```python
from build123d import *

# Parameters (mm, degrees)
SKETCH_1_R        = 110
SKETCH_1_R_2      = 3
SKETCH_1_R_3      = 90
EXTRUDE_1_DEPTH   = 10
SKETCH_1_R_4      = 80
SKETCH_1_R_5      = 75
EXTRUDE_1_2_DEPTH = 10
SKETCH_1_3_R      = 90
SKETCH_1_3_R_2    = 80
SKETCH_1_3_R_3    = 75
EXTRUDE_2_DEPTH   = 5
SKETCH_2_R        = 90
SKETCH_2_R_2      = 80
EXTRUDE_4_DEPTH   = 5


with BuildPart() as part:
    # Sketch 1 → Extrude 1 (new body)
    with BuildSketch(Plane(origin=(0, 0, 0), x_dir=(1, 0, 0), z_dir=(0, 1, 0))):
        with Locations(Location((0, 0, 0), (0, 0, 270))):
            Circle(SKETCH_1_R)
        with Locations(Location((-38.268343237, 92.387953251, 0), (0, 0, 270))):
            Circle(SKETCH_1_R_2, mode=Mode.SUBTRACT)
        with Locations(Location((-70.710678119, 70.710678119, 0), (0, 0, 270))):
            Circle(SKETCH_1_R_2, mode=Mode.SUBTRACT)
        with Locations(Location((-92.387953251, 38.268343237, 0), (0, 0, 270))):
            Circle(SKETCH_1_R_2, mode=Mode.SUBTRACT)
        with Locations(Location((-100, 0, 0), (0, 0, 270))):
            Circle(SKETCH_1_R_2, mode=Mode.SUBTRACT)
        with Locations(Location((-92.387953251, -38.268343237, 0), (0, 0, 270))):
            Circle(SKETCH_1_R_2, mode=Mode.SUBTRACT)
        with Locations(Location((-70.710678119, -70.710678119, 0), (0, 0, 270))):
            Circle(SKETCH_1_R_2, mode=Mode.SUBTRACT)
        with Locations(Location((-38.268343237, -92.387953251, 0), (0, 0, 270))):
            Circle(SKETCH_1_R_2, mode=Mode.SUBTRACT)
        with Locations(Location((0, -100, 0), (0, 0, 270))):
            Circle(SKETCH_1_R_2, mode=Mode.SUBTRACT)
        with Locations(Location((38.268343237, -92.387953251, 0), (0, 0, 270))):
            Circle(SKETCH_1_R_2, mode=Mode.SUBTRACT)
        with Locations(Location((70.710678119, -70.710678119, 0), (0, 0, 270))):
            Circle(SKETCH_1_R_2, mode=Mode.SUBTRACT)
        with Locations(Location((92.387953251, -38.268343237, 0), (0, 0, 270))):
            Circle(SKETCH_1_R_2, mode=Mode.SUBTRACT)
        with Locations(Location((100, 0, 0), (0, 0, 270))):
            Circle(SKETCH_1_R_2, mode=Mode.SUBTRACT)
        with Locations(Location((92.387953251, 38.268343237, 0), (0, 0, 270))):
            Circle(SKETCH_1_R_2, mode=Mode.SUBTRACT)
        with Locations(Location((70.710678119, 70.710678119, 0), (0, 0, 270))):
            Circle(SKETCH_1_R_2, mode=Mode.SUBTRACT)
        with Locations(Location((38.268343237, 92.387953251, 0), (0, 0, 270))):
            Circle(SKETCH_1_R_2, mode=Mode.SUBTRACT)
        with Locations(Location((0, 100, 0), (0, 0, 270))):
            Circle(SKETCH_1_R_2, mode=Mode.SUBTRACT)
        with Locations(Location((0, 0, 0), (0, 0, 270))):
            Circle(SKETCH_1_R_3, mode=Mode.SUBTRACT)
    extrude(amount=EXTRUDE_1_DEPTH)



with BuildPart() as body_2:
    # Sketch 1 → Extrude 1 2 (new body)
    with BuildSketch(Plane(origin=(0, 0, 0), x_dir=(1, 0, 0), z_dir=(0, 1, 0))):
        with Locations(Location((0, 0, 0), (0, 0, 270))):
            Circle(SKETCH_1_R_4)
        with Locations(Location((0, 0, 0), (0, 0, 270))):
            Circle(SKETCH_1_R_5, mode=Mode.SUBTRACT)
    extrude(amount=EXTRUDE_1_2_DEPTH)


with BuildPart() as part_1:
    add(part.part)

    add(body_2.part)  # Extrude 2 merges body 2
    # Sketch 1_3 → Extrude 2 (add)
    # profile 1 of 2: a face of its own
    with BuildSketch(Plane(origin=(0, 0, 0), x_dir=(1, 0, 0), z_dir=(0, 1, 0))):
        with Locations(Location((0, 0, 0), (0, 0, 270))):
            Circle(SKETCH_1_3_R)
        with Locations(Location((0, 0, 0), (0, 0, 270))):
            Circle(SKETCH_1_3_R_2, mode=Mode.SUBTRACT)
    # profile 2 of 2: a face of its own
    with BuildSketch(Plane(origin=(0, 0, 0), x_dir=(1, 0, 0), z_dir=(0, 1, 0))):
        with Locations(Location((0, 0, 0), (0, 0, 270))):
            Circle(SKETCH_1_3_R_3)
    extrude(amount=EXTRUDE_2_DEPTH)

    # Sketch 2 → Extrude 4 (add)
    with BuildSketch(Plane(origin=(0, 5, 0), x_dir=(1, 0, 0), z_dir=(0, 1, 0))):
        Circle(SKETCH_2_R)
        Circle(SKETCH_2_R_2, mode=Mode.SUBTRACT)
    extrude(amount=EXTRUDE_4_DEPTH)

    # Sweep 1: sweep along a path in Sketch 5
    with BuildLine(Plane(origin=(0, 5, 0), x_dir=(1, 0, 0), z_dir=(0, 1, 0))) as sweep_1_path:
        CenterArc((0, 0), 85, 0, 360)
    # Sketch 4 → Sweep 1 (sweep, cut)
    with BuildSketch(Plane.XY):
        with BuildLine():
            Line((90, 10), (80, 10))
            ThreePointArc((80, 10), (85, 5), (90, 10))
        make_face()
    sweep(path=sweep_1_path.line, mode=Mode.SUBTRACT)


solid = part_1.part
```
Input: part model. Units: mm. Frame: model coordinates. A direction names the side the tool comes from. Give positions to 0.01 mm unless a question says otherwise; leave off trailing zeros. Loops run counter-clockwise (first coordinate to the right, second up) from the corner with the lowest first, then second, coordinate; pieces in that order, holes last. Notation, with made-up numbers: (75.5, -32.75) -> (81.5, -32.75) arc R27 cw to (81.5, -3.75) -> close; hole circle Ø9 at (-30, 25.5). An arc over 180 degrees is marked (long way). Use a Markdown table: item, result.
Q1. Section query D-D, the plane x = 100. Return the cut outline in (y, z), plus the area to 3 significant figures.
Entries:
| item | result |
|---|---|
| outline | (0, -45.83) -> (10, -45.83) -> (10, -3) -> (0, -3) -> close; (0, 3) -> (10, 3) -> (10, 45.83) -> (0, 45.83) -> close |
| area | 857 mm² |
Q2. Access query for faces 1 (the flat face through (1, 5, -1)), 2 (the cylindrical face through (-68.18, 4.93, -69.1)). Directions: +Z, -Z, +X, -X, +Y, -Y. A direction counts if a zero-diameter tool reaches every point of the face in a straight line with its end or side. Return the directions, or none.
Entries:
| item | result |
|---|---|
| face 1 | +Y |
| face 2 | +Y, -Y |
Q3. Section query A-A, the plane y = 7.5. State how many separate pieces and enclosed holes the cut face has, plus the area to 3 significant figures.
Entries:
| item | result |
|---|---|
| separate pieces | 2 |
| enclosed holes | 18 |
| area | 15,300 mm² |
Q4. Section query B-B, the plane x = 0. Return the cut outline in (y, z), plus the area to 3 significant figures.
Entries:
| item | result |
|---|---|
| outline | (0, -110) -> (10, -110) -> (10, -103) -> (0, -103) -> close; (0, -97) -> (10, -97) -> (10, -90) arc R5 cw to (10, -80) -> (10, -75) -> (5, -75) -> (5, 75) -> (10, 75) -> (10, 80) arc R5 cw to (10, 90) -> (10, 97) -> (0, 97) -> close; (0, 103) -> (10, 103) -> (10, 110) -> (0, 110) -> close |
| area | 1,250 mm² |
Q5. Ray query, probe 1 along X at (y, z) = (3.25, 0); probe 2 along X at (y, z) = (9.75, 51); probe 3 along X at (y, z) = (7, -91.5). Return the intervals inside material, ascending. Write a range as from..to.
Entries:
| item | result |
|---|---|
| probe 1 | x = -110..-103, -97..97, 103..110 |
| probe 2 | x = -97.46..-74.15, -61.64..-54.99, 54.99..61.64, 74.15..97.46 |
| probe 3 | x = -61.06..-41.13, -35.4..35.4, 41.13..61.06 |
Q6. First-contact query: P1, Ø4, axis at x = 41.5, z = -54, coming from the +Y side; P2, Ø1, axis at x = 8.5, y = 6.5, coming from the +Z side; P3, Ø1.5, axis at x = -31.5, y = 2, coming from the -Z side. Flat tips, straight axial feed; report the tip coordinate or a pass-through.
Entries:
| item | result |
|---|---|
| P1 | stops at y = 5 |
| P2 | stops at z = 109.71 |
| P3 | stops at z = -105.61 |
Q7. Section query C-C, the plane z = 0. Return the cut outline in (x, y).
Entries:
| item | result |
|---|---|
| outline | (-110, 0) -> (-103, 0) -> (-103, 10) -> (-110, 10) -> close; (-97, 0) -> (97, 0) -> (97, 10) -> (90, 10) arc R5 cw to (80, 10) -> (75, 10) -> (75, 5) -> (-75, 5) -> (-75, 10) -> (-80, 10) arc R5 cw to (-90, 10) -> (-97, 10) -> close; (103, 0) -> (110, 0) -> (110, 10) -> (103, 10) -> close |
